```python
from build123d import *

# Parameters (mm, degrees)
F0_W     = 400
F0_H     = 500
F1_DEPTH = 3
F2_W     = 10
F2_H     = 3
F2_W_2   = 20
F3_DEPTH = 3
F4_W     = 20
F4_H     = 3
F5_DEPTH = 25


with BuildPart() as f1:
    # F0 (on Right) → F1 (new body)
    with BuildSketch(Plane.YZ):
        Rectangle(F0_W, F0_H)
    extrude(amount=F1_DEPTH)

    # F2 (on face) → F3 (join, through all)
    with BuildSketch(Plane.YZ.offset(3)):
        with Locations((-195, 251.5)):
            Rectangle(F2_W, F2_H)
        with Locations((-160, 251.5)):
            Rectangle(F2_W_2, F2_H)
        with Locations((-120, 251.5)):
            Rectangle(F2_W_2, F2_H)
        with Locations((-80, 251.5)):
            Rectangle(F2_W_2, F2_H)
        with Locations((-40, 251.5)):
            Rectangle(F2_W_2, F2_H)
        with Locations((0, 251.5)):
            Rectangle(F2_W_2, F2_H)
        with Locations((40, 251.5)):
            Rectangle(F2_W_2, F2_H)
        with Locations((80, 251.5)):
            Rectangle(F2_W_2, F2_H)
        with Locations((120, 251.5)):
            Rectangle(F2_W_2, F2_H)
        with Locations((160, 251.5)):
            Rectangle(F2_W_2, F2_H)
        with Locations((195, 251.5)):
            Rectangle(F2_W, F2_H)
        with Locations((-120, -251.5)):
            Rectangle(F2_W_2, F2_H)
        with Locations((-160, -251.5)):
            Rectangle(F2_W_2, F2_H)
        with Locations((-80, -251.5)):
            Rectangle(F2_W_2, F2_H)
        with Locations((0, -251.5)):
            Rectangle(F2_W_2, F2_H)
        with Locations((160, -251.5)):
            Rectangle(F2_W_2, F2_H)
        with Locations((80, -251.5)):
            Rectangle(F2_W_2, F2_H)
        with Locations((195, -251.5)):
            Rectangle(F2_W, F2_H)
        with Locations((40, -251.5)):
            Rectangle(F2_W_2, F2_H)
        with Locations((-195, -251.5)):
            Rectangle(F2_W, F2_H)
        with Locations((-40, -251.5)):
            Rectangle(F2_W_2, F2_H)
        with Locations((120, -251.5)):
            Rectangle(F2_W_2, F2_H)
    extrude(amount=-F3_DEPTH)

    # F4 (on face) → F5 (cut)
    with BuildSketch(Plane.YZ.offset(3)):
        with Locations((-180, -151.5)):
            Rectangle(F4_W, F4_H)
        with Locations((-140, -151.5)):
            Rectangle(F4_W, F4_H)
        with Locations((-100, -151.5)):
            Rectangle(F4_W, F4_H)
        with Locations((-60, -151.5)):
            Rectangle(F4_W, F4_H)
        with Locations((-20, -151.5)):
            Rectangle(F4_W, F4_H)
        with Locations((20, -151.5)):
            Rectangle(F4_W, F4_H)
        with Locations((60, -151.5)):
            Rectangle(F4_W, F4_H)
        with Locations((100, -151.5)):
            Rectangle(F4_W, F4_H)
        with Locations((140, -151.5)):
            Rectangle(F4_W, F4_H)
        with Locations((180, -151.5)):
            Rectangle(F4_W, F4_H)
    extrude(amount=-F5_DEPTH, mode=Mode.SUBTRACT)


solid = f1.part
```
Design review of the part built by this model. Coordinates are the model's own, in mm. Coordinates: 2 decimals unless noted, no trailing zeros. Order: outer loops, then holes, each group sorted by start corner. A loop starts at its lowest first (then second) coordinate and runs counter-clockwise, first axis right, second up. Notation, with made-up numbers: (13, -11) - (65, -11) arc R19 cw to (65, 14) - close; hole circle Ø1 at (-2, 5). An arc over 180 degrees is marked (long way). Answer in a Markdown table with one row per item.
(1) Wall thickness on line 1 along Z through (x, y) = (0.85, -65): over which ranges is the line inside the solid? List them lowest first. Write a range as from..to.
Checked values:
| item | result |
|---|---|
| line 1 | -250..-153, -150..250 |
(2) Clearance check with flat-ended pins moving along their axes: pin 1 (0.9 mm diameter, centred on x = 1, y = -56.5, fed in from -Z); pin 2 (5 mm diameter, centred on y = 156.5, z = -189, fed in from -X); pin 3 (1.5 mm diameter, centred on x = 1, y = -96.5, fed in from +Z). State where each tip first meets the part, or that it passes through.
Checked values:
| item | result |
|---|---|
| pin 1 | z = -250 |
| pin 2 | x = 0 |
| pin 3 | z = 250 |
(3) Consider section A-A on y = -98. State the section outline as (x, z) points, plus the area to 3 significant figures.
Checked values:
| item | result |
|---|---|
| outline | (0, -250) - (3, -250) - (3, -153) - (0, -153) - close; (0, -150) - (3, -150) - (3, 250) - (0, 250) - close |
| area | 1,490 mm^2 |
